The listing builds one solid part. Answer for the finished solid, in the listing's coordinates (mm). A direction names the side the tool comes from. Round coordinates to 2 decimals unless told otherwise and drop trailing zeros. Loops run counter-clockwise (first coordinate to the right, second up) from the corner with the lowest first, then second, coordinate; pieces in that order, holes last. Notation, with made-up numbers: M 37,-9 L 66,-9 A20 cw 66,16 Z; hole C 63.25,41 d1. An arc over 180 degrees is marked long. Answer as a JSON object with one key per item and string values.
```python
from build123d import *

# Parameters (mm, degrees)
BOSS_EXTRUDE1_DEPTH = 3
SKETCH2_W           = 28
SKETCH2_H           = 28
BOSS_EXTRUDE2_DEPTH = 1.5
SKETCH3_W           = 25
SKETCH3_H           = 25
BOSS_EXTRUDE3_DEPTH = 3.5


with BuildPart() as part:
    # Sketch1 → Boss-Extrude1 (new body)
    with BuildSketch(Plane.XY):
        Polygon((-166.007283518, 36), (-186.007283518, 36), (-188.007283518, 34), (-188.007283518, 14), (-186.007283518, 12), (-166.007283518, 12), (-164.007283518, 14), (-164.007283518, 34), align=None)
    extrude(amount=BOSS_EXTRUDE1_DEPTH)

    # Sketch2 → Boss-Extrude2 (add)
    with BuildSketch(Plane.XY.offset(3)):
        with Locations((-176.007283518, 24)):
            Rectangle(SKETCH2_W, SKETCH2_H)
    extrude(amount=BOSS_EXTRUDE2_DEPTH)

    # Sketch3 → Boss-Extrude3 (add)
    with BuildSketch(Plane.XY.offset(4.5)):
        with Locations((-176.007283518, 24)):
            Rectangle(SKETCH3_W, SKETCH3_H)
    extrude(amount=BOSS_EXTRUDE3_DEPTH)


solid = part.part
```
Item 1: The part is cut by section A-A (x = -175). Give the vertices of the cut face in (y, z).
Values follow:
{"outline": "M 10,3 L 12,3 L 12,0 L 36,0 L 36,3 L 38,3 L 38,4.5 L 36.5,4.5 L 36.5,8 L 11.5,8 L 11.5,4.5 L 10,4.5 Z"}
Item 2: The part is cut by section C-C (z = 7). Give the vertices of the cut face in (x, y).
Values follow:
{"outline": "M -188.51,11.5 L -163.51,11.5 L -163.51,36.5 L -188.51,36.5 Z"}
Item 3: Straight lines are drawn through the part: line 1 (Y direction, x = -170.25, z = 6.5); line 2 (X direction, y = 12, z = 6.5); line 3 (Z direction, x = -164.75, y = 12.75). For each, find the intervals that lie inside material, in ascending order.
Values follow:
{"line 1": "11.5 to 36.5", "line 2": "-188.51 to -163.51", "line 3": "3 to 8"}
Item 4: Which of the six approach directions +Z, -Z, +X, -X, +Y, -Y give full straight-line access (tool end or side, diameter ignored) to faces 1 (the face through (-186.993, 35.014, 1.479)), 2 (the face through (-165.02, 12.99, 1.48)), 3 (the face through (-187.02, 13.01, 1.48))?
Values follow:
{"face 1": "-Z, -X, +Y", "face 2": "-Z, +X, -Y", "face 3": "-Z, -X, -Y"}
Item 5: The part is cut by section B-B (y = 33.5). Give the vertices of the cut face in (x, z), then the cut area to 4 significant figures.
Values follow:
{"outline": "M -190.01,3 L -188.01,3 L -188.01,0 L -164.01,0 L -164.01,3 L -162.01,3 L -162.01,4.5 L -163.51,4.5 L -163.51,8 L -188.51,8 L -188.51,4.5 L -190.01,4.5 Z", "area": "201.5 mm^2"}
Item 6: Flat-ended cylindrical pins translate along their axes: P1, Ø0.9, axis at x = -174, z = 2, coming from the -Y side; P2, Ø0.9, axis at y = 22, z = 2, coming from the +X side; P3, Ø4, axis at y = 20, z = 7, coming from the +X side. Find the tip coordinate at first contact, or state that the pin passes through.
Values follow:
{"P1": "y = 12", "P2": "x = -164.01", "P3": "x = -163.51"}
